```python
from build123d import *

# Parameters (mm, degrees)
F0_W     = 42
F0_H     = 120
F1_DEPTH = 8
F2_W     = 42
F2_H     = 120
F2_W_2   = 30
F2_H_2   = 100
F3_DEPTH = 25
F4_W     = 15
F4_H     = 10
F5_DEPTH = 25
F6_DEPTH = 1
F7_DEPTH = 1
F8_R     = 1.75
F8_R_2   = 4.25
F9_DEPTH = 25


with BuildPart() as f1:
    # F0 (on Top) → F1 (new body)
    with BuildSketch(Plane.XY):
        Rectangle(F0_W, F0_H)
    extrude(amount=F1_DEPTH)

    # F2 (on face) → F3 (cut)
    with BuildSketch(Plane.XY.offset(8)):
        Rectangle(F2_W, F2_H)
        Rectangle(F2_W_2, F2_H_2, mode=Mode.SUBTRACT)
    extrude(amount=-F3_DEPTH, mode=Mode.SUBTRACT)

    # F4 (on face) → F5 (cut)
    with BuildSketch(Plane.XY.offset(8)):
        with Locations((-7.5, 45)):
            Rectangle(F4_W, F4_H)
        with Locations((7.5, -45)):
            Rectangle(F4_W, F4_H)
    extrude(amount=-F5_DEPTH, mode=Mode.SUBTRACT)

    # F6 (add): a face of the model
    f6_faces = [f1.faces().sort_by_distance(p)[0] for p in [
        (-7.5, 40, 4),
    ]]
    extrude(f6_faces, amount=F6_DEPTH)

    # F7 (add): a face of the model
    f7_faces = [f1.faces().sort_by_distance(p)[0] for p in [
        (7.5, -40, 4),
    ]]
    extrude(f7_faces, amount=F7_DEPTH)

    # F8 (on face) → F9 (cut)
    with BuildSketch(Plane.XY.offset(8)):
        with Locations((9, 46)):
            Circle(F8_R)
        with Locations((-9, -46)):
            Circle(F8_R)
        with Locations((0, 26)):
            Circle(F8_R_2)
        with Locations((0, -26)):
            Circle(F8_R_2)
    extrude(amount=-F9_DEPTH, mode=Mode.SUBTRACT)


solid = f1.part
```
CAD build for the part. Positions are in the model's coordinates, mm. A direction names the side the tool comes from. Round coordinates to 2 decimals unless told otherwise and drop trailing zeros. Loops run counter-clockwise (first coordinate to the right, second up) from the corner with the lowest first, then second, coordinate; pieces in that order, holes last. Notation, with made-up numbers: (86, -18.75) - (106, -18.75) arc R30 cw to (106, 7.25) - close; hole circle Ø7 at (47.5, 83). An arc over 180 degrees is marked (long way). Return JSON: item names as keys, results as strings. Group by question number.
Q1. Band-saw the part on C-C on x = -9. Give the cut face in (y, z).
Q2. Band-saw the part on B-B on z = 2. Give the cut face in (x, y), plus the area to 3 significant figures.
Q3. Tool access for faces 1 (the face through (7, -41, 4)), 2 (the face through (0, 45, 4)), 3 (the face through (-9.38, -47.71, 4.06)): list every direction of +Z, -Z, +X, -X, +Y, -Y with a clear straight run to the whole face (end or side of a thin tool).
Q4. Two-plate mould, pull along Y, no slides. Class faces 4 (the face through (-0.553, 30.214, 4.056)), 5 (the face through (-8, 41, 4)), 6 (the face through (0, -46, 4)): +Y half, -Y half, draft (parallel to the pull), parting line (faces both ways), or undercut.
Q5. Band-saw the part on D-D on x = -2.5. Give the cut face in (y, z), plus the area to 3 significant figures.
Q6. Flat gauge pins, fed straight in: pin 1 Ø1.5 at (x, z) = (6, 6) entering from -Y; pin 2 Ø2 at (x, y) = (-9, -46) entering from -Z; pin 3 Ø4 at (x, z) = (-5, 5) entering from +Y. Where does each tip first touch, or does it go through?
Q7. Band-saw the part on A-A on y = -46. Give the cut face in (x, z), plus the area to 3 significant figures.
Q8. Drill centre lines: line 1 along Y through (x, z) = (0.5, 1); line 2 along Y through (x, z) = (9, 4.5); line 3 along Y through (x, z) = (-9, 4.5). Where is each one in solid material? Low to high. Write a range as [from, to].
Solutions:
{
 "1": {"outline": "(-50, 0) - (-47.75, 0) - (-47.75, 8) - (-50, 8) - close; (-44.25, 0) - (41, 0) - (41, 8) - (-44.25, 8) - close"},
 "2": {"outline": "(-15, -50) - (0, -50) - (0, -41) - (15, -41) - (15, 50) - (0, 50) - (0, 41) - (-15, 41) - close; hole circle Ø3.5 at (-9, -46); hole circle Ø8.5 at (0, -26); hole circle Ø8.5 at (0, 26); hole circle Ø3.5 at (9, 46)", "area": "2,600 mm^2"},
 "3": {"face 1": "+Z, -Z, +X, -Y", "face 2": "+Z, -Z, -X, +Y", "face 3": "+Z, -Z"},
 "4": {"face 4": "undercut", "face 5": "+Y half", "face 6": "draft"},
 "5": {"outline": "(-50, 0) - (-29.44, 0) - (-29.44, 8) - (-50, 8) - close; (-22.56, 0) - (22.56, 0) - (22.56, 8) - (-22.56, 8) - close; (29.44, 0) - (41, 0) - (41, 8) - (29.44, 8) - close", "area": "618 mm^2"},
 "6": {"pin 1": "stops at y = -41", "pin 2": "passes through", "pin 3": "stops at y = 41"},
 "7": {"outline": "(-15, 0) - (-10.75, 0) - (-10.75, 8) - (-15, 8) - close; (-7.25, 0) - (0, 0) - (0, 8) - (-7.25, 8) - close", "area": "92.0 mm^2"},
 "8": {"line 1": "y = [-41, -30.22], [-21.78, 21.78], [30.22, 50]", "line 2": "y = [-41, 44.25], [47.75, 50]", "line 3": "y = [-50, -47.75], [-44.25, 41]"}
}
